Input: part model. Units: mm. Frame: model coordinates. Round coordinates to 2 decimals unless told otherwise and drop trailing zeros. Loops run counter-clockwise (first coordinate to the right, second up) from the corner with the lowest first, then second, coordinate; pieces in that order, holes last. Notation, with made-up numbers: (-26, 54.25) -> (-16, 54.25) arc R26 cw to (-16, 74.25) -> close; hole circle Ø1 at (22.5, 23). An arc over 180 degrees is marked (long way). Answer as a JSON object with one key per item and string values.
Autodesk Inventor part; units mm, degrees
ref_plane "YZ Plane" through (0, 0, 0) normal (1, 0, 0) x (0, 1, 0)
ref_plane "XZ Plane" through (0, 0, 0) normal (0, 1, 0) x (-1, 0, 0)
ref_plane "XY Plane" through (0, 0, 0) normal (0, 0, 1) x (1, 0, 0)
ref_plane "Work Plane1" through (0, 0, 0) normal (0, 0, 1) x (0, -1, 0)
sketch "Sketch1" plane through (0, 0, 0) normal (0, 0, 1) x (0, -1, 0)
  line L0 (-450.85, 82.6732) -> (0, 82.6732) construction
  line L1 (0, -5) -> (-450.85, -5) construction
  line L2 (-450.85, -5) -> (-450.85, 82.6732)
  line L3 (0, 82.6732) -> (0, -5)
  line L4 (0, -5) -> (-450.85, -5)
  circle A0 centre (-444.5, 22.86) radius 1.7 construction
  circle A1 centre (-444.5, 54.8132) radius 1.7 construction
  circle A2 centre (-252.8255, 65.525) radius 1.9304 construction
  circle A3 centre (-210.0251, 141.725) radius 1.9304 construction
  circle A4 centre (-6.35, 54.8132) radius 1.7 construction
  circle A5 centre (-6.35, 22.86) radius 1.7 construction
  circle A6 centre (-94.9, 14.5) radius 1.7 construction
  circle A7 centre (-349.219, 14.5) radius 1.7 construction
  circle A8 centre (-444.5, 22.86) radius 1.65
  circle A9 centre (-444.5, 54.8132) radius 1.65
  circle A10 centre (-349.219, 14.5) radius 1.65
  circle A11 centre (-210.0251, 141.725) radius 1.65
  circle A12 centre (-94.9, 14.5) radius 1.65
  circle A13 centre (-6.35, 54.8132) radius 1.65
  circle A14 centre (-6.35, 22.86) radius 1.65
  circle A15 centre (-78.0653, 61.3428) radius 1.905
  line L5 (-78.0653, 61.3428) -> (-78.0653, 23.2428) construction
  line L6 (-78.0653, 23.2428) -> (-39.9653, 23.2428) construction
  line L7 (-39.9653, 23.2428) -> (-39.9653, 61.3428) construction
  circle A16 centre (-78.0653, 23.2428) radius 1.905
  circle A17 centre (-39.9653, 23.2428) radius 1.905
  circle A18 centre (-39.9653, 61.3428) radius 1.905
  line L8 (-450.85, 15.32) -> (-438.15, 15.32) construction
  line L9 (-246.7618, 27.8034) -> (-231.5218, 27.8034)
  line L10 (-231.5218, 27.8034) -> (-231.5218, 37.9634)
  line L11 (-231.5218, 37.9634) -> (-246.7618, 37.9634)
  line L12 (-246.7618, 37.9634) -> (-246.7618, 27.8034)
  line L13 (-345.7194, 77.136) -> (-345.7194, 60.0672)
  line L14 (-345.7194, 60.0672) -> (-256.8194, 60.0672)
  line L15 (-256.8194, 60.0672) -> (-256.8194, 77.136)
  line L16 (-450.85, 82.6732) -> (-345.7194, 82.6732)
  line L17 (-450.85, 82.6732) -> (0, 82.6732)
  circle A19 centre (-162.5271, 23.6214) radius 1.65
  circle A20 centre (-244.1194, 68.6016) radius 1.1906
  line L18 (-345.7194, 77.136) -> (-256.8194, 77.136)
  circle A21 centre (-358.4194, 68.6016) radius 1.1906
  line L19 (-301.2694, 60.0672) -> (-301.2694, 77.136) construction
  line L20 (-323.85, 17.86) -> (-270.51, 17.86)
  line L21 (-270.51, 17.86) -> (-270.51, 43.26)
  line L22 (-270.51, 43.26) -> (-323.85, 43.26)
  line L23 (-323.85, 43.26) -> (-323.85, 17.86)
  circle A22 centre (-264.16, 30.56) radius 1.1906
  circle A23 centre (-330.2, 30.56) radius 1.1906
  point P0 (0, 0)
  dimension "M3Clearance" = 3.3
  dimension "d1" = 3.3
  dimension "d2" = 3.3
  dimension "d4" = 3.3
  dimension "d5" = 3.3
  dimension "d6" = 3.3
  dimension "d7" = 3.3
  dimension "Number6Clearance" = 3.81
  dimension "d9" = 38.1
  dimension "d10" = 38.1
  dimension "d11" = 38.1
  dimension "d12" = 3.81
  dimension "d13" = 3.81
  dimension "d14" = 3.81
  dimension "d21" = 12.7
  dimension "d22" = 20.32
  dimension "d24" = 15.24
  dimension "d25" = 10.16
  dimension "d26" = 22.606
  dimension "d36" = 3.3
  dimension "d37" = 47.498
  dimension "d38" = 59.0518
  dimension "d39" = 59.0518
  dimension "Number6WoodScrewPilot" = 2.3813
  dimension "d41" = 8.5344
  dimension "d42" = 12.7
  dimension "d43" = 5.5372
  dimension "d44" = 17.0688
  dimension "d45" = 2.3813
  dimension "d46" = 8.5344
  dimension "d47" = 12.7
  dimension "d48" = 149.5806
  dimension "d49" = 44.45
  dimension "d50" = 127
  dimension "d51" = 53.34
  dimension "d52" = 22.86
  dimension "d53" = 25.4
  dimension "d54" = 2.3813
  dimension "d55" = 12.7
  dimension "d56" = 6.35
  dimension "d57" = 2.3813
  dimension "d58" = 6.35
  dimension "d59" = 12.7
extrude "Extrusion1" add sketch "Sketch1" along normal blind 5 contours L2 L16 L17 L3 L4
sketch "Sketch4" plane through (0, 0, 5) normal (0, 0, 1) x (1, 0, 0)
  circle A0 centre (54.8132, 95.25) radius 1.7 construction
  circle A1 centre (22.86, 95.25) radius 1.7 construction
  circle A2 centre (54.8132, 368.3) radius 1.7 construction
  circle A3 centre (22.86, 368.3) radius 1.7 construction
  circle A4 centre (22.86, 95.25) radius 1.65
  circle A5 centre (54.8132, 95.25) radius 1.65
  circle A6 centre (22.86, 368.3) radius 1.65
  circle A7 centre (54.8132, 368.3) radius 1.65
  point P0 (0, 0)
  dimension "d60" = 3.3
  dimension "d61" = 3.3
  dimension "d62" = 3.3
  dimension "d63" = 3.3
extrude "Extrusion3" cut sketch "Sketch4" against normal blind 5
equation "\"d1\" = M3Clearance"
equation "\"d2\" = M3Clearance"
equation "\"d4\" = M3Clearance"
equation "\"d5\" = M3Clearance"
equation "\"d6\" = M3Clearance"
equation "\"d7\" = M3Clearance"
equation "\"d12\" = Number6Clearance"
equation "\"d13\" = Number6Clearance"
equation "\"d14\" = Number6Clearance"
equation "\"d21\" = d55"
equation "\"d36\" = M3Clearance"
equation "\"d39\" = d38"
equation "\"d41\" = 0.5 * d44"
equation "\"d45\" = Number6WoodScrewPilot"
equation "\"d46\" = d41"
equation "\"d47\" = d42"
equation "\"d54\" = Number6WoodScrewPilot"
equation "\"d55\" = 0.5 * d53"
equation "\"d57\" = Number6WoodScrewPilot"
equation "\"d58\" = d56"
equation "\"d60\" = M3Clearance"
equation "\"d61\" = M3Clearance"
equation "\"d62\" = M3Clearance"
equation "\"d63\" = M3Clearance"
properties part number "top of drivetrain 2"
1) Section B-B, the plane z = 4. Count the separate pieces of the cut face and the enclosed holes in it, plus the area to 3 significant figures.
Output:
{"separate pieces": "1", "enclosed holes": "22", "area": "36,300 mm^2"}
2) Ray query, probe 1 along X at (y, z) = (6.35, 1.1); probe 2 along X at (y, z) = (95.25, 1.55); probe 3 along X at (y, z) = (323, 3.4). Return the intervals inside material, ascending.
Output:
{"probe 1": "x = -5 to 21.21, 24.51 to 53.16, 56.46 to 82.67", "probe 2": "x = -5 to 12.89, 16.11 to 21.21, 24.51 to 53.16, 56.46 to 82.67", "probe 3": "x = -5 to 17.86, 43.26 to 60.07, 77.14 to 82.67"}
3) Section A-A, the plane y = 293.5. Output: boundary loops of the cut face in (x, z), plus the area to 3 significant figures.
Output:
{"outline": "(-5, 0) -> (17.86, 0) -> (17.86, 5) -> (-5, 5) -> close; (43.26, 0) -> (60.07, 0) -> (60.07, 5) -> (43.26, 5) -> close; (77.14, 0) -> (82.67, 0) -> (82.67, 5) -> (77.14, 5) -> close", "area": "226 mm^2"}
